Autodesk Inventor part; units mm, degrees
ref_plane "YZ Plane" through (0, 0, 0) normal (1, 0, 0) x (0, 1, 0)
ref_plane "XZ Plane" through (0, 0, 0) normal (0, 1, 0) x (-1, 0, 0)
ref_plane "XY Plane" through (0, 0, 0) normal (0, 0, 1) x (1, 0, 0)
sketch "Sketch1" plane through (0, 0, 0) normal (0, 0, 1) x (1, 0, 0)
  circle A0 centre (0, 0) radius 7
  dimension "d0" = 14
extrude "Extrusion1" add sketch "Sketch1" along normal blind 7
sketch "Sketch2" plane through (0, 0, 7) normal (0, 0, 1) x (1, 0, 0)
  circle A0 centre (0, 0) radius 5
  dimension "d3" = 10
extrude "Extrusion2" add sketch "Sketch2" along normal blind 31
chamfer "Chamfer1" distance 1 angle 45 1 edges at (-5, 0, 38)
properties part number "bolt"
Check sheet for the modelled part. Datum: model origin and axes. Units: mm. A direction names the side the tool comes from. Coordinates: 2 decimals unless noted, no trailing zeros. Order: outer loops, then holes, each group sorted by start corner. A loop starts at its lowest first (then second) coordinate and runs counter-clockwise, first axis right, second up. Notation, with made-up numbers: (12, 37) -> (29, 37) arc R23 ccw to (29, 59) -> close; hole circle Ø9 at (5, -27). An arc over 180 degrees is marked (long way). Write item = value, one per line. Start each with the question number.
1) Go/stop test with flat-tipped pins: P1, Ø3, axis at y = 0.5, z = 32, coming from the -X side; P2, Ø1, axis at x = -1.5, z = 25.5, coming from the -Y side; P3, Ø1, axis at y = 1.5, z = 19, coming from the -X side. Record where each tip stops, or that it passes through.
2) Cross-section at A-A (x = 0). Enter the section's corners in (y, z), then the cut area to 3 significant figures.
3) Material ranges on L1, parallel to Y at x = 0, z = 8; L2, parallel to Z at x = -3.25, y = -4.25; L3, parallel to X at y = 4, z = 31, recorded low to high.
4) Cross-section at C-C (z = 29). Enter the section's corners in (x, y).
5) Access from +Z, -Z, +X, -X, +Y, -Y to the whole of each face (thin tool, end or side, straight path). Record for faces 1 (the cylindrical face through (-1.08, 4.88, 21.79)), 2 (the flat face through (0, 0, 38)).
Ans:
q1.P1 = -5
q1.P2 = -4.9
q1.P3 = -4.9
q2.outline = (-7, 0) -> (7, 0) -> (7, 7) -> (5, 7) -> (5, 37) -> (4, 38) -> (-4, 38) -> (-5, 37) -> (-5, 7) -> (-7, 7) -> close
q2.area = 407 mm²
q3.L1 = -5 to 5
q3.L2 = 0 to 7
q3.L3 = -3 to 3
q4.outline = circle Ø10 at (0, 0)
q5.face_1 = +Z
q5.face_2 = +Z, +X, -X, +Y, -Y
